The listing builds one solid part. Answer for the finished solid, in the listing's coordinates (mm). A direction names the side the tool comes from. Coordinates: 2 decimals unless noted, no trailing zeros. Loops run counter-clockwise (first coordinate to the right, second up) from the corner with the lowest first, then second, coordinate; pieces in that order, holes last. Notation, with made-up numbers: M 85.25,56 L 102.25,56 A21 cw 102.25,75 Z; hole C -30,42.5 d4. An arc over 180 degrees is marked long. Return JSON: item names as keys, results as strings. Group by question number.
1. Section B-B (x = 0) is taken. Write down the section's boundary in (y, z).
2. The mould has two halves that part along X. Classify faces 4 (the face through (-9.5, 0.07, 1.97)), 5 (the face through (-5, 0, -7.2)), 6 (the face through (1.116, -5.028, -5.423)): pulls with the +X half, pulls with the -X half, needs draft (parallel to the pull), parting line crosses it, or undercut.
3. Section D-D (y = -8) is taken. Write down the section's boundary in (x, z).
4. Section C-C (z = -7.75) is taken. Write down the section's boundary in (x, y), then the cut area to 3 significant figures.
5. Section A-A (y = 0) is taken. Write down the section's boundary in (x, z).
6. Given P1, Ø0.5, axis at x = -4, y = -1, coming from the -Z side; P2, Ø5, axis at x = -5, z = 1.5, coming from the +Y side; P3, Ø1, axis at x = 4, z = -9, coming from the -Y side; P4, Ø5, axis at x = 0, y = 0, coming from the -Z side, each flat-ended and moving along its own axis, determine where each tip first touches the part or whether it passes through.
7. Straight lines are drawn through the part: L1, parallel to Y at x = 0, z = 1.55; L2, parallel to X at y = -1, z = 1.75; L3, parallel to Z at x = -2.5, y = -7. For each, find the intervals that lie inside material, in ascending order. Write a range as from..to.
8. Which of the six approach directions +Z, -Z, +X, -X, +Y, -Y give full straight-line access (tool end or side, diameter ignored) to faces 1 (the face through (2, -5, 0)), 2 (the face through (6.5, 0.07, 1.97)), 3 (the face through (-4, 1.8, -9))?
```python
from build123d import *

# Parameters (mm, degrees)
SKETCH_1_R               = 11
SKETCH_1_R_2             = 1.5
EXTRUDE_1_DEPTH          = 4
SKETCH_2_R               = 5.15
EXTRUDE_2_DEPTH          = 11
SKETCH_3_R               = 4
CUT_EXTRUDE_1_DEPTH      = 1
CUT_EXTRUDE_1_DEPTH_BACK = 16
SKETCH_6_W               = 3.8
SKETCH_6_H               = 3.6
CUT_EXTRUDE_2_DEPTH      = 12
CUT_EXTRUDE_2_DEPTH_BACK = 12


with BuildPart() as part:
    # 草图1 → 凸台-拉伸1 (new body)
    with BuildSketch(Plane.XY):
        Circle(SKETCH_1_R)
        with Locations((-8, 0)):
            Circle(SKETCH_1_R_2, mode=Mode.SUBTRACT)
        with Locations((0, 8)):
            Circle(SKETCH_1_R_2, mode=Mode.SUBTRACT)
        with Locations((8, 0)):
            Circle(SKETCH_1_R_2, mode=Mode.SUBTRACT)
        with Locations((0, -8)):
            Circle(SKETCH_1_R_2, mode=Mode.SUBTRACT)
    extrude(amount=EXTRUDE_1_DEPTH)

    # 草图2 → 凸台-拉伸2 (add)
    with BuildSketch(Plane(origin=(0, 0, 0), x_dir=(-1, 0, 0), z_dir=(0, 0, -1))):
        Circle(SKETCH_2_R)
    extrude(amount=EXTRUDE_2_DEPTH)

    # 草图3 → 切除-拉伸1 (cut, two sides)
    with BuildSketch(Plane(origin=(0, 0, -11), x_dir=(-1, 0, 0), z_dir=(0, 0, -1))) as cut_extrude_1_sk:
        Circle(SKETCH_3_R)
    extrude(amount=CUT_EXTRUDE_1_DEPTH, mode=Mode.SUBTRACT)
    extrude(cut_extrude_1_sk.sketch, amount=-CUT_EXTRUDE_1_DEPTH_BACK, mode=Mode.SUBTRACT)

    # 草图6 → 切除-拉伸2 (cut, two sides)
    with BuildSketch(Plane.ZY) as cut_extrude_2_sk:
        with Locations((-9.1, 0)):
            Rectangle(SKETCH_6_W, SKETCH_6_H)
    extrude(amount=CUT_EXTRUDE_2_DEPTH, mode=Mode.SUBTRACT)
    extrude(cut_extrude_2_sk.sketch, amount=-CUT_EXTRUDE_2_DEPTH_BACK, mode=Mode.SUBTRACT)


solid = part.part
```
Worked out:
{
 "1": {"outline": "M -11,0 L -9.5,0 L -9.5,4 L -11,4 Z; M -6.5,0 L -5.15,0 L -5.15,-11 L -4,-11 L -4,4 L -6.5,4 Z; M 4,-11 L 5.15,-11 L 5.15,0 L 6.5,0 L 6.5,4 L 4,4 Z; M 9.5,0 L 11,0 L 11,4 L 9.5,4 Z"},
 "2": {"face 4": "undercut", "face 5": "needs draft", "face 6": "parting line crosses it"},
 "3": {"outline": "M -7.55,0 L -1.5,0 L -1.5,4 L -7.55,4 Z; M 1.5,0 L 7.55,0 L 7.55,4 L 1.5,4 Z"},
 "4": {"outline": "M -4.83,-1.8 A5.15 ccw 4.83,-1.8 L 3.57,-1.8 A4 cw -3.57,-1.8 Z; M -4.83,1.8 L -3.57,1.8 A4 cw 3.57,1.8 L 4.83,1.8 A5.15 ccw Z", "area": "24.5 mm^2"},
 "5": {"outline": "M -11,0 L -9.5,0 L -9.5,4 L -11,4 Z; M -6.5,0 L -5.15,0 L -5.15,-7.2 L -4,-7.2 L -4,4 L -6.5,4 Z; M 4,-7.2 L 5.15,-7.2 L 5.15,0 L 6.5,0 L 6.5,4 L 4,4 Z; M 9.5,0 L 11,0 L 11,4 L 9.5,4 Z"},
 "6": {"P1": "z = -7.2", "P2": "y = 10.71", "P3": "y = -3.78", "P4": "through"},
 "7": {"L1": "-11..-9.5, -6.5..-4, 4..6.5, 9.5..11", "L2": "-10.95..-9.12, -6.88..-3.87, 3.87..6.88, 9.12..10.95", "L3": "0..4"},
 "8": {"face 1": "-Z", "face 2": "+Z, -Z", "face 3": "-Z, +X, -X"}
}
